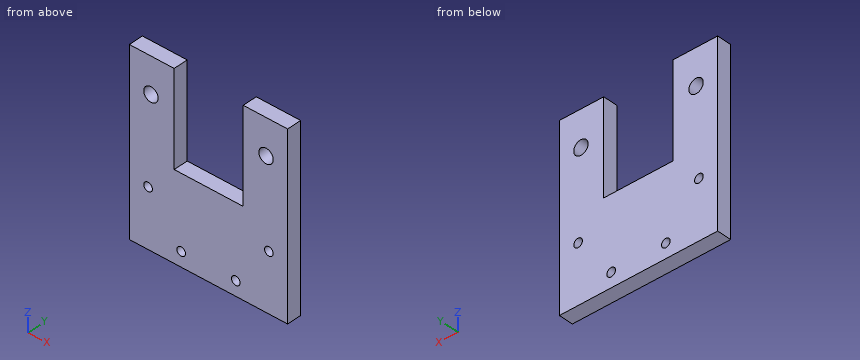
from build123d import *

# Parameters (mm, degrees)
SKETCH1_W           = 65
SKETCH1_H           = 100
BOSS_EXTRUDE1_DEPTH = 5
SKETCH3_R           = 1.5
SKETCH3_R_2         = 2.5
CUT_EXTRUDE2_DEPTH  = 5
SKETCH5_W           = 24
SKETCH5_H           = 70
CUT_EXTRUDE4_DEPTH  = 5
SKETCH6_W           = 65
SKETCH6_H           = 10
CUT_EXTRUDE5_DEPTH  = 5
SKETCH7_W           = 20.576460324
SKETCH7_H           = 27.703955477
CUT_EXTRUDE6_DEPTH  = 5
SKETCH8_W           = 20.423539676
SKETCH8_H           = 27.703955477
CUT_EXTRUDE7_DEPTH  = 5
CUT_EXTRUDE8_DEPTH  = 5
SKETCH10_W          = 5
SKETCH10_H          = 62.296044523
CUT_EXTRUDE9_DEPTH  = 5


with BuildPart() as part:
    # Sketch1 → Boss-Extrude1 (new body)
    with BuildSketch(Plane(origin=(0, 0, 0), x_dir=(1, 0, 0), z_dir=(0, 1, 0))):
        Rectangle(SKETCH1_W, SKETCH1_H)
    extrude(amount=BOSS_EXTRUDE1_DEPTH)

    # Sketch3 → Cut-Extrude2 (cut)
    with BuildSketch(Plane(origin=(0, 5, 0), x_dir=(1, 0, 0), z_dir=(0, 1, 0))):
        with Locations(Location((-21, 30, 0), (0, 0, 270))):
            Circle(SKETCH3_R)
        with Locations(Location((21, 30, 0), (0, 0, 270))):
            Circle(SKETCH3_R)
        with Locations(Location((-9.5, 45, 0), (0, 0, 270))):
            Circle(SKETCH3_R)
        with Locations(Location((9.5, 45, 0), (0, 0, 270))):
            Circle(SKETCH3_R)
        with Locations(Location((-20, 0, 0), (0, 0, 270))):
            Circle(SKETCH3_R_2)
        with Locations(Location((20, 0, 0), (0, 0, 270))):
            Circle(SKETCH3_R_2)
    extrude(amount=-CUT_EXTRUDE2_DEPTH, mode=Mode.SUBTRACT)

    # Sketch5 → Cut-Extrude4 (cut)
    with BuildSketch(Plane(origin=(0, 5, 0), x_dir=(1, 0, 0), z_dir=(0, 1, 0))):
        with Locations((0.076460324, -15)):
            Rectangle(SKETCH5_W, SKETCH5_H)
    extrude(amount=-CUT_EXTRUDE4_DEPTH, mode=Mode.SUBTRACT)

    # Sketch6 → Cut-Extrude5 (cut)
    with BuildSketch(Plane(origin=(0, 5, 0), x_dir=(1, 0, 0), z_dir=(0, 1, 0))):
        with Locations((0, -45)):
            Rectangle(SKETCH6_W, SKETCH6_H)
    extrude(amount=-CUT_EXTRUDE5_DEPTH, mode=Mode.SUBTRACT)

    # Sketch7 → Cut-Extrude6 (cut)
    with BuildSketch(Plane(origin=(0, 5, 0), x_dir=(1, 0, 0), z_dir=(0, 1, 0))):
        with Locations((-22.211769838, -26.148022261)):
            Rectangle(SKETCH7_W, SKETCH7_H)
    extrude(amount=-CUT_EXTRUDE6_DEPTH, mode=Mode.SUBTRACT)

    # Sketch8 → Cut-Extrude7 (cut)
    with BuildSketch(Plane(origin=(0, 5, 0), x_dir=(1, 0, 0), z_dir=(0, 1, 0))):
        with Locations((22.288230162, -26.148022261)):
            Rectangle(SKETCH8_W, SKETCH8_H)
    extrude(amount=-CUT_EXTRUDE7_DEPTH, mode=Mode.SUBTRACT)

    # Sketch9 → Cut-Extrude8 (cut)
    with BuildSketch(Plane(origin=(0, 5, 0), x_dir=(1, 0, 0), z_dir=(0, 1, 0))):
        Polygon((-27.5, 34.801314728), (-27.5, 50), (-32.5, 50), (-32.5, -12.296044523), (-27.5, -12.296044523), (-27.5, 18.851977738), align=None)
    extrude(amount=-CUT_EXTRUDE8_DEPTH, mode=Mode.SUBTRACT)

    # Sketch10 → Cut-Extrude9 (cut)
    with BuildSketch(Plane(origin=(0, 5, 0), x_dir=(1, 0, 0), z_dir=(0, 1, 0))):
        with Locations((30, 18.851977739)):
            Rectangle(SKETCH10_W, SKETCH10_H)
    extrude(amount=-CUT_EXTRUDE9_DEPTH, mode=Mode.SUBTRACT)


solid = part.part
The model under review builds one solid part; all positions refer to its coordinate system, in mm. Give positions to 0.01 mm unless a question says otherwise; leave off trailing zeros. Write each loop counter-clockwise with the first axis right and the second up, starting at its lowest first coordinate (ties: lowest second). Pieces come first, ordered by that corner, then holes. Notation, with made-up numbers: M -30.5,18.5 L 22.5,18.5 A10 ccw 22.5,37.5 Z; hole C 13,11.25 d10. An arc over 180 degrees is marked long. One line per question, with ' | ' between items. Start each with the question number.
Item 1: For pin 1 (2.5 mm diameter, centred on x = 0, y = 3, fed in from +Z), flat-tipped, find the tip position at first contact; note if it passes through.
Item 2: We need section D-D on z = -4. Write out the cut boundary in (x, y).
Item 3: We need section C-C on y = 1.6. Write out the cut boundary in (x, z), plus the area to 3 significant figures.
Item 4: Wall thickness on line 1 (X direction, y = 3.7, z = -30); line 2 (X direction, y = 2.8, z = -17.5); line 3 (X direction, y = 0.5, z = -29): over which ranges is each line inside the solid? List them lowest first. Write a range as from..to.
Item 5: We need section B-B on x = 9.5. Write out the cut boundary in (y, z), plus the area to 3 significant figures.
Item 6: We need section A-A on z = -30. Write out the cut boundary in (x, y), plus the area to 3 significant figures.
Results found:
1) pin 1: stops at z = -20
2) outline: M -27.5,0 L -11.92,0 L -11.92,5 L -27.5,5 Z; M 12.08,0 L 27.5,0 L 27.5,5 L 12.08,5 Z
3) outline: M -27.5,-50 L 27.5,-50 L 27.5,12.3 L 12.08,12.3 L 12.08,-20 L -11.92,-20 L -11.92,12.3 L -27.5,12.3 Z; hole C -21,-30 d3; hole C -20,0 d5; hole C -9.5,-45 d3; hole C 9.5,-45 d3; hole C 20,0 d5; hole C 21,-30 d3 | area: 2,580 mm2
4) line 1: x = -27.5..-22.5, -19.5..19.5, 22.5..27.5 | line 2: x = -27.5..-11.92, 12.08..27.5 | line 3: x = -27.5..-22.12, -19.88..19.88, 22.12..27.5
5) outline: M 0,-50 L 5,-50 L 5,-46.5 L 0,-46.5 Z; M 0,-43.5 L 5,-43.5 L 5,-20 L 0,-20 Z | area: 135 mm2
6) outline: M -27.5,0 L -22.5,0 L -22.5,5 L -27.5,5 Z; M -19.5,0 L 19.5,0 L 19.5,5 L -19.5,5 Z; M 22.5,0 L 27.5,0 L 27.5,5 L 22.5,5 Z | area: 245 mm2
